Autodesk Inventor part; units mm, degrees
ref_plane "YZ Plane" through (0, 0, 0) normal (1, 0, 0) x (0, 1, 0)
ref_plane "XZ Plane" through (0, 0, 0) normal (0, 1, 0) x (-1, 0, 0)
ref_plane "XY Plane" through (0, 0, 0) normal (0, 0, 1) x (1, 0, 0)
sketch "Sketch1" plane through (0, 0, 0) normal (0, 1, 0) x (-1, 0, 0)
  line L0 (-175, 200) -> (175, 200)
  line L1 (175, 200) -> (175, -200)
  line L2 (175, -200) -> (-175, -200)
  line L3 (-175, -200) -> (-175, 200)
  line L4 (-175, 200) -> (175, -200) construction
  line L5 (175, 200) -> (-175, -200) construction
  point P0 (0, 0)
  dimension "d0" = 350
  dimension "d1" = 400
extrude "Extrusion1" add sketch "Sketch1" along normal blind 30
fillet "Fillet1" radius 30 4 edges at (0, 30, 200) (-175, 30, 0) (175, 30, 0) (0, 30, -200)
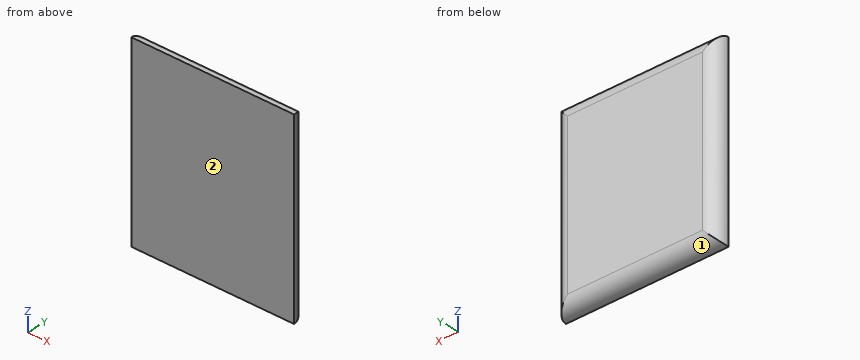
Build history of the part. All positions in model axes, mm. Face numbers are marked on the shaded views. Coordinates: 2 decimals unless noted, no trailing zeros. Order: outer loops, then holes, each group sorted by start corner. A loop starts at its lowest first (then second) coordinate and runs counter-clockwise, first axis right, second up. Notation, with made-up numbers: (59, -19) - (72, -19) arc R22 cw to (72, 13) - close; hole circle Ø4 at (51.25, 2). An arc over 180 degrees is marked (long way). Write each question's results on one line, items separated by ' | '. Start each with the question number.
Item 1: Flat gauge pins, fed straight in: pin 1 (8 mm diameter, centred on y = 9, z = 113, fed in from +X); pin 2 (3 mm diameter, centred on x = 21, y = 16, fed in from +Z); pin 3 (4 mm diameter, centred on x = -38, y = 20.5, fed in from +Z). Where does each tip first touch, or does it go through?
Item 2: Band-saw the part on C-C on y = 15.75. Write the cut outline in (x, z), and give its area (3 significant figures).
Item 3: Mould opens along Z. For the marked faces 1 and 2 say: released by +Z, released by -Z, zero draft, split by the parting line, or undercut.
Item 4: Wall check: probe 1 along Y at (x, z) = (145.5, 39.5); probe 2 along Y at (x, z) = (-8, -173); probe 3 along X at (y, z) = (5.75, -16). Give the ranges that are in metal, low to high. Write a range as [from, to].
Numbers:
1) pin 1: x = 174.58 | pin 2: z = 196.26 | pin 3: z = 193.62
2) outline: (-170.53, -195.53) - (170.53, -195.53) - (170.53, 195.53) - (-170.53, 195.53) - close | area: 133,000 mm^2
3) face 1: released by -Z | face 2: zero draft
4) probe 1: [0, 30] | probe 2: [0, 29.85] | probe 3: [-174.44, 174.44]
